Geometry: see drawing. Coordinates: mm, zero at the bounding-box minimum. Coordinates: 2 decimals unless noted, no trailing zeros. Order: outer loops, then holes, each group sorted by start corner. A loop starts at its lowest first (then second) coordinate and runs counter-clockwise, first axis right, second up.
Item 1: Section B-B on y = 4. Return the cut outline in (x, z).
Item 2: Ray query, line 1 (Z direction, x = 4, y = 4.25); line 2 (X direction, y = 2, z = 10.5); line 3 (Z direction, x = 1.5, y = 3.5). Return the intervals inside material, ascending.
Item 3: Section C-C on z = 27. Return the cut outline in (x, y), then the cut area to 3 significant figures.
Item 4: Contact query for flat-ended pins moving along their axis: P1, Ø1.5, axis at x = 5, z = 15, coming from the +Y side; P2, Ø3, axis at x = 6, z = 16, coming from the +Y side; P3, Ø1, axis at x = 5, z = 13.5, coming from the -Y side. Output: stop coordinate, or through.
Item 5: Mould query, pull axis X, two halves, no side actions, for the marked faces 1, 2 and 3. Classes: released by +X, released by -X, zero draft, split by the parting line, or undercut.
Item 6: Section A-A on x = 4. Return the cut outline in (y, z), then the cut area to 3 significant figures.
Item 7: Section D-D on z = 11. Return the cut outline in (x, y).
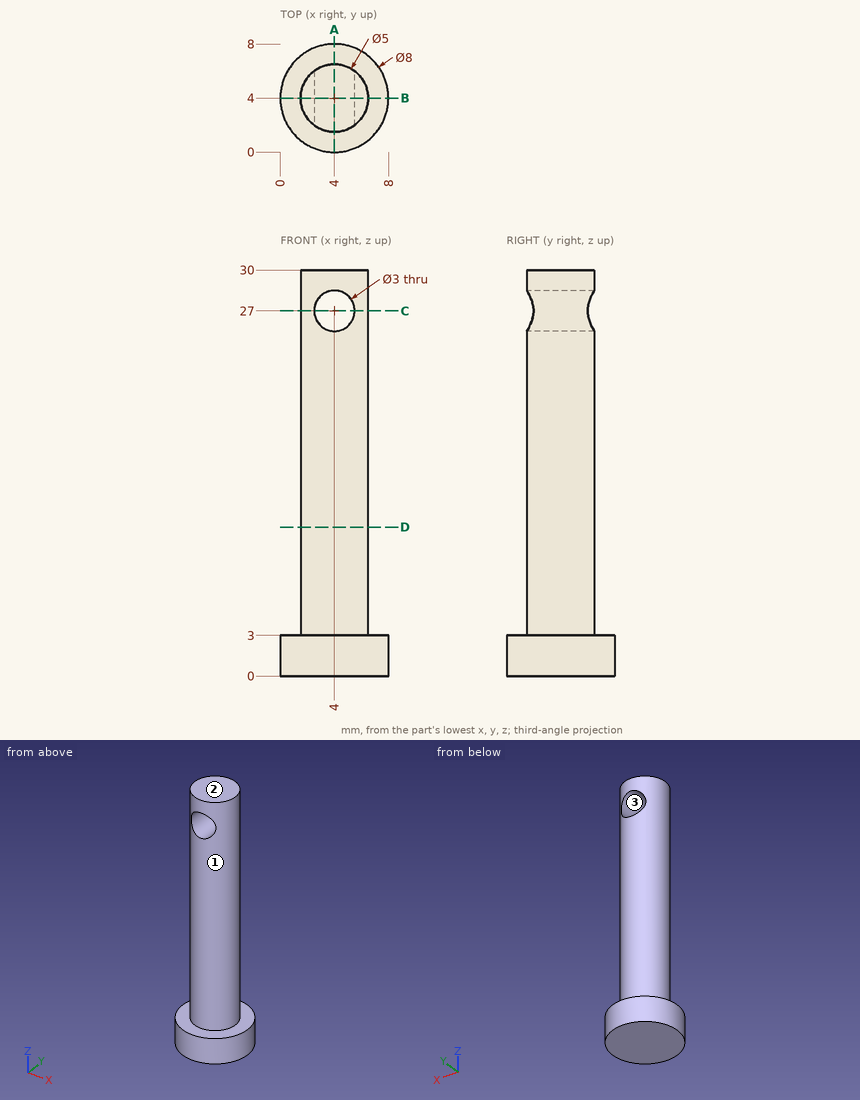
Answer list:
1. outline: (0, 0) - (8, 0) - (8, 3) - (6.5, 3) - (6.5, 30) - (1.5, 30) - (1.5, 3) - (0, 3) - close; hole circle Ø3 at (4, 27)
2. line 1: z = 0 to 25.5, 28.5 to 30
2. line 2: x = 2.5 to 5.5
2. line 3: z = 0 to 3
3. outline: (2.5, 2) - (2.5, 6) arc R2.5 ccw to start; (5.5, 2) arc R2.5 ccw to (5.5, 6) - close
3. area: 5.59 mm2
4. P1: stops at y = 6.49
4. P2: stops at y = 6.45
4. P3: stops at y = 1.55
5. face 1: split by the parting line
5. face 2: zero draft
5. face 3: undercut
6. outline: (0, 0) - (8, 0) - (8, 3) - (6.5, 3) - (6.5, 25.5) - (1.5, 25.5) - (1.5, 3) - (0, 3) - close; (1.5, 28.5) - (6.5, 28.5) - (6.5, 30) - (1.5, 30) - close
6. area: 144 mm2
7. outline: circle Ø5 at (4, 4)
